Could you check a few things on this model? Use its own coordinates, in mm. Face numbers are marked on the shaded views. A direction names the side the tool comes from. Give positions to 0.01 mm unless a question says otherwise; leave off trailing zeros. Loops run counter-clockwise (first coordinate to the right, second up) from the corner with the lowest first, then second, coordinate; pieces in that order, holes last. Notation, with made-up numbers: (18.5, 87) -> (61.5, 87) arc R28 ccw to (61.5, 110) -> close; hole circle Ø9 at (-37.5, 24). An arc over 180 degrees is marked (long way). Write each question's results on one line, items separated by ' | '. Start each with the question number.
Q1. Will these pins go through, and if not, where does the flat tip stop? P1, Ø2, axis at x = -7.5, y = -33.5, coming from the +Z side; P2, Ø3, axis at x = -7, y = -35, coming from the -Z side; P3, Ø1, axis at x = -11, y = -49.5, coming from the -Z side; P4, Ø3.5, axis at x = -9.5, z = 0.5, coming from the +Y side.
Q2. If we section it at B-B, the plane z = 0: List the corners of the cut face in (x, y) for me.
Q3. Which directions (+Z, -Z, +X, -X, +Y, -Y) give clear straight access to the entire face, cutting with the end or side of a thin tool? Please do the marked faces 4 and 5.
Q4. If I drill on line 1 along Y through (x, z) = (-8.5, 2.25); line 2 along Z through (x, y) = (-10, -36); line 3 along Z through (x, y) = (-8.75, -32.75), over which ranges is the centre line in solid material (lowest first)?
Q5. If we section it at A-A, the plane y = -47.5: List the corners of the cut face in (x, z) for me.
Q6. We'd pull the mould along X, two halves only. Please class the marked faces 1, 2 and 3: released by +X, released by -X, zero draft, split by the parting line, or undercut.
Autodesk Inventor part; units mm, degrees
ref_plane "YZ Plane" through (0, 0, 0) normal (1, 0, 0) x (0, 1, 0)
ref_plane "XZ Plane" through (0, 0, 0) normal (0, 1, 0) x (-1, 0, 0)
ref_plane "XY Plane" through (0, 0, 0) normal (0, 0, 1) x (1, 0, 0)
sketch "Sketch1" plane through (0, 0, 0) normal (0, 0, 1) x (1, 0, 0)
  line L0 (-9.9228, -30) -> (-13.5328, -30)
  line L1 (-13.5328, -30) -> (-13.5328, -26)
  line L2 (-13.5328, -26) -> (-9.9228, -26)
  line L3 (-9.9228, -26) -> (-9.9228, -30)
  line L4 (-9.9228, -30) -> (-9.9228, -55)
  line L5 (-9.9228, -55) -> (-11.9228, -55)
  line L6 (-11.9228, -55) -> (-11.9228, -30)
  point P0 (0, 0)
  dimension "d0" = 3.61
  dimension "d1" = 4
  dimension "d3" = 2
  dimension "d16" = 25
revolve "Revolution1" add sketch "Sketch1" angle 360 about axis through (-9.9228, -30, 0) along (0, -1, 0)
chamfer "Chamfer1" distance 0.4 angle 45 1 edges at (-6.3128, -26, 0)
sketch "Boceto2" plane through (-9.9228, -26, 0) normal (0, 1, 0) x (1, 0, 0)
  line L0 (1.1641, -1.3443) -> (-0.5821, -1.6803)
  line L1 (-0.5821, -1.6803) -> (-1.7462, -0.336)
  line L2 (-1.7462, -0.336) -> (-1.1641, 1.3443)
  line L3 (-1.1641, 1.3443) -> (0.5821, 1.6803)
  line L4 (0.5821, 1.6803) -> (1.7462, 0.336)
  line L5 (1.7462, 0.336) -> (1.1641, -1.3443)
  point P0 (9.9228, 0)
  point P1 (0, 0)
  dimension "d11" = 3.08
extrude "Extrusión1" cut sketch "Boceto2" against normal blind 2
thread "Rosca1"
properties part number "Tornillo Allen cabeza cilindrica M4x25mm"
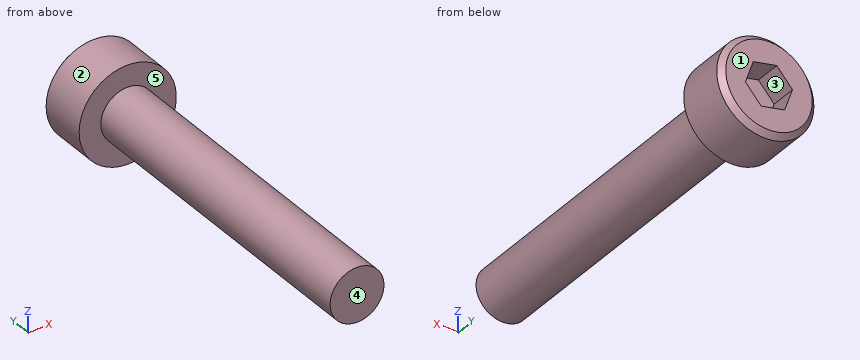
Final values:
1) P1: stops at z = 1.41 | P2: stops at z = -1.41 | P3: stops at z = -1.91 | P4: stops at y = -26
2) outline: (-13.53, -30) -> (-11.92, -30) -> (-11.92, -55) -> (-7.92, -55) -> (-7.92, -30) -> (-6.31, -30) -> (-6.31, -26.4) -> (-6.71, -26) -> (-8.29, -26) -> (-8.29, -28) -> (-11.55, -28) -> (-11.55, -26) -> (-13.13, -26) -> (-13.53, -26.4) -> close
3) face 4: +Z, -Z, +X, -X, -Y | face 5: -Y
4) line 1: y = -30 to -26 | line 2: z = -2 to 2 | line 3: z = -1.62 to 1.62
5) outline: circle Ø4 at (-9.92, 0)
6) face 1: zero draft | face 2: split by the parting line | face 3: undercut
